Design review of the part shown in the three views and the two pictorial views. Dimensions are in mm from the part's minimum x, y and z. A direction names the side the tool comes from. Round coordinates to 2 decimals unless told otherwise and drop trailing zeros. Order: outer loops, then holes, each group sorted by start corner. A loop starts at its lowest first (then second) coordinate and runs counter-clockwise, first axis right, second up. Notation, with made-up numbers: (-8.5, 24.25) - (0.5, 24.25) arc R24 cw to (0.5, 59.25) - close; hole circle Ø7 at (-10.5, -25.75). An arc over 180 degrees is marked (long way). One line per question, with ' | ' between items. Start each with the question number.
Item 1: Add section D-D on z = 5.5. State the section outline as (x, y) points.
Item 2: Tool access review of the marked faces 1 and 2: name each direction out of +Z, -Z, +X, -X, +Y, -Y from which nothing blocks a thin tool from reaching the whole face with its end or side.
Item 3: For L1, parallel to Z at x = 0.5, y = 2; L2, parallel to Y at x = 3.5, z = 16; L3, parallel to X at y = 2, z = 17, list the stretches that pass through material, from the lowest coordinate up. Write a range as [from, to].
Item 4: Insertion check: pin 1 Ø1 at (x, z) = (5.5, 16) entering from -Y; pin 2 Ø2 at (y, z) = (3.5, 6) entering from -X; pin 3 Ø3 at (y, z) = (1, 9) entering from +X. Each pin has a flat end and moves straight along its axis. Give the tip position at first contact, or say it passes through.
Item 5: Add section A-A on x = 2. State the section outline as (y, z) points, and give its area (3 significant figures).
Item 6: Add section B-B on y = 3.5. State the section outline as (x, z) points.
Item 7: Add section C-C on z = 14.25. State the section outline as (x, y) points.
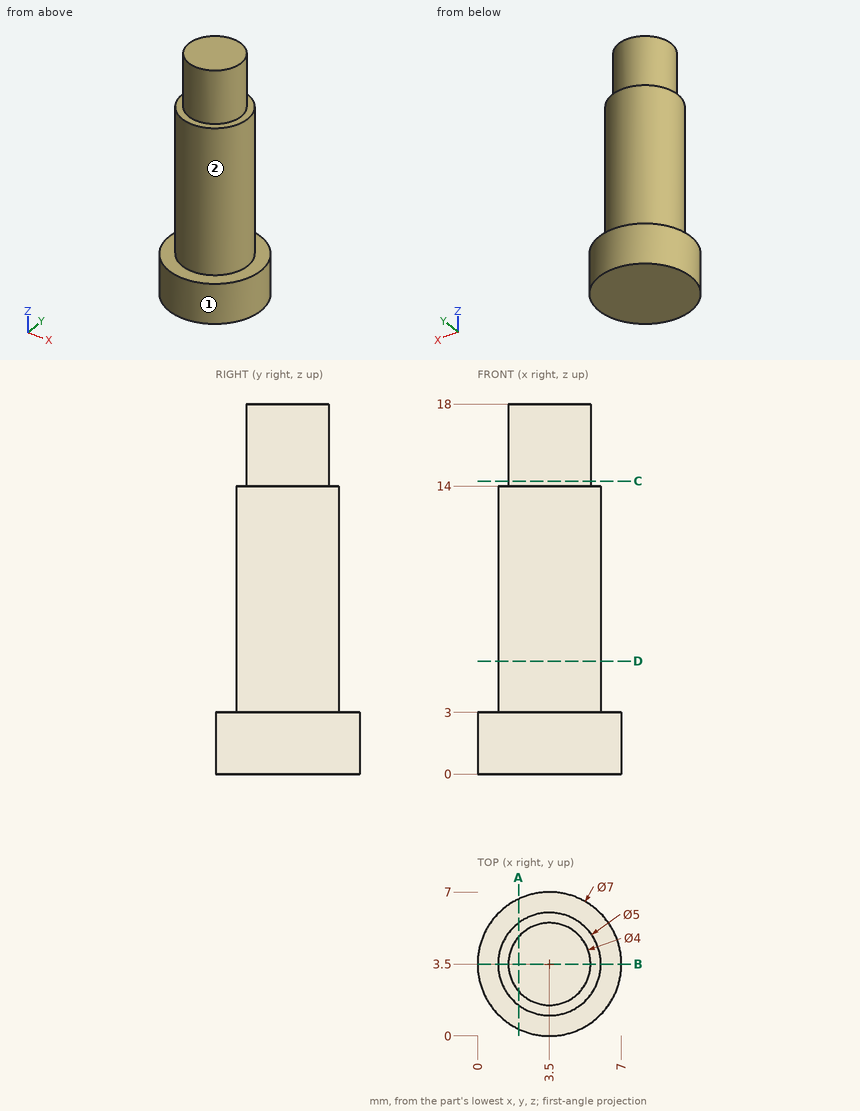
Determined:
1) outline: circle Ø5 at (3.5, 3.5)
2) face 1: +Z, -Z | face 2: +Z
3) L1: [0, 3] | L2: [1.5, 5.5] | L3: [2.18, 4.82]
4) pin 1: y = 2.18 | pin 2: x = 1 | pin 3: x = 5.79
5) outline: (0.34, 0) - (6.66, 0) - (6.66, 3) - (5.5, 3) - (5.5, 14) - (4.82, 14) - (4.82, 18) - (2.18, 18) - (2.18, 14) - (1.5, 14) - (1.5, 3) - (0.34, 3) - close | area: 73.6 mm2
6) outline: (0, 0) - (7, 0) - (7, 3) - (6, 3) - (6, 14) - (5.5, 14) - (5.5, 18) - (1.5, 18) - (1.5, 14) - (1, 14) - (1, 3) - (0, 3) - close
7) outline: circle Ø4 at (3.5, 3.5)
